from build123d import *

# Parameters (mm, degrees)
F0_W     = 50
F0_H     = 30
F1_DEPTH = 5
F2_W     = 30
F2_H     = 30
F3_DEPTH = 1
F4_SIZE  = 2
F5_R     = 2.5
F6_DEPTH = 25
F7_R     = 0.5
F8_DEPTH = 25


with BuildPart() as f1:
    # F0 (on Top) → F1 (new body)
    with BuildSketch(Plane.XY):
        Rectangle(F0_W, F0_H)
    extrude(amount=F1_DEPTH)

    # F2 (on face) → F3 (cut)
    with BuildSketch(Plane.XY.offset(5)):
        Rectangle(F2_W, F2_H)
    extrude(amount=-F3_DEPTH, mode=Mode.SUBTRACT)

    # F4
    f4_edges = [f1.edges().sort_by_distance(p)[0] for p in [
        (-25, 15, 2.5),
        (-25, -15, 2.5),
        (25, -15, 2.5),
        (25, 15, 2.5),
    ]]
    chamfer(f4_edges, length=F4_SIZE)

    # F5 (on face) → F6 (cut)
    with BuildSketch(Plane.XY.offset(5)):
        with Locations((-20, 10)):
            Circle(F5_R)
        with Locations((-20, -10)):
            Circle(F5_R)
        with Locations((20, -10)):
            Circle(F5_R)
        with Locations((20, 10)):
            Circle(F5_R)
    extrude(amount=-F6_DEPTH, mode=Mode.SUBTRACT)

    # F7 (on face) → F8 (cut)
    with BuildSketch(Plane.XY.offset(4)):
        with Locations((-4.5, 0)):
            Circle(F7_R)
        with Locations((4.5, 0)):
            Circle(F7_R)
    extrude(amount=-F8_DEPTH, mode=Mode.SUBTRACT)


solid = f1.part
Could you check a few things on this model? Use its own coordinates, in mm. A direction names the side the tool comes from. Give positions to 0.01 mm unless a question says otherwise; leave off trailing zeros. Write each loop counter-clockwise with the first axis right and the second up, starting at its lowest first coordinate (ties: lowest second). Pieces come first, ordered by that corner, then holes. Notation, with made-up numbers: (80, 21) -> (111, 21) arc R24 ccw to (111, 34) -> close; hole circle Ø1 at (39, -31.5). An arc over 180 degrees is marked (long way). Answer as CSV lines item,"result". Start each with the question number.
(1) Please list where these lines run through material, in increasing order: line 1 (Y direction, x = 20, z = 3.85); line 2 (Y direction, x = -4.5, z = 2.6); line 3 (Y direction, x = 18.5, z = 4.7).
(2) If we section it at A-A, the plane x = 4.5: Write out the boundary of the cut face in (y, z).
(3) If we section it at B-B, the plane x = 22: Write out the boundary of the cut face in (y, z).
(4) If we mould it in two halves opening along X, with no side actions, what happens to faces 1 (the face through (-22, -11.5, 2.5)), 2 (the face through (24, 14, 2)), 3 (the face through (20, 0, 5))? For each: +X half, -X half, draft (parallel to the pull), parting line (faces both ways), or undercut.
(5) If we section it at C-C, the plane y = -8.5: Write out the boundary of the cut face in (x, z).
(6) I'm going to push flat-ended pins straight in: pin 1 Ø3 at (x, y) = (7.5, 11.5) entering from +Z; pin 2 Ø1 at (x, y) = (-18.5, 9.5) entering from +Z. Where does each tip first touch, or does it pass through?
(7) If we section it at D-D, the plane z = 1.05: Write out the boundary of the cut face in (x, y), and give its area (3 significant figures).
(8) Which directions (+Z, -Z, +X, -X, +Y, -Y) give clear straight access to the entire face, cutting with the end or side of a thin tool? Please do faces 4 (the face through (4, 0, 2)), 5 (the face through (15, -0.2, 4.5)).
Answer list:
1,line 1,"-15 to -12.5, -7.5 to 7.5, 12.5 to 15"
1,line 2,"-15 to -0.5, 0.5 to 15"
1,line 3,"-15 to -12, -8 to 8, 12 to 15"
2,outline,"(-15, 0) -> (-0.5, 0) -> (-0.5, 4) -> (-15, 4) -> close; (0.5, 0) -> (15, 0) -> (15, 4) -> (0.5, 4) -> close"
3,outline,"(-15, 0) -> (-11.5, 0) -> (-11.5, 5) -> (-15, 5) -> close; (-8.5, 0) -> (8.5, 0) -> (8.5, 5) -> (-8.5, 5) -> close; (11.5, 0) -> (15, 0) -> (15, 5) -> (11.5, 5) -> close"
4,face 1,"undercut"
4,face 2,"+X half"
4,face 3,"draft"
5,outline,"(-25, 0) -> (-22, 0) -> (-22, 5) -> (-25, 5) -> close; (-18, 0) -> (18, 0) -> (18, 5) -> (15, 5) -> (15, 4) -> (-15, 4) -> (-15, 5) -> (-18, 5) -> close; (22, 0) -> (25, 0) -> (25, 5) -> (22, 5) -> close"
6,pin 1,"z = 4"
6,pin 2,"through"
7,outline,"(-25, -13) -> (-23, -15) -> (23, -15) -> (25, -13) -> (25, 13) -> (23, 15) -> (-23, 15) -> (-25, 13) -> close; hole circle Ø5 at (-20, -10); hole circle Ø5 at (-20, 10); hole circle Ø1 at (-4.5, 0); hole circle Ø1 at (4.5, 0); hole circle Ø5 at (20, -10); hole circle Ø5 at (20, 10)"
7,area,"1,410 mm^2"
8,face 4,"+Z, -Z"
8,face 5,"+Z, +Y, -Y"
